from build123d import *

# Parameters (mm, degrees)
SCHIZZO1_R                    = 8
ESTRUSIONE_ESTRUSIONE1_DEPTH  = 30
SCHIZZO2_R                    = 2.5
TAGLIO_ESTRUSIONE1_DEPTH      = 33.062439084
SCHIZZO3_R                    = 4
TAGLIO_ESTRUSIONE2_DEPTH      = 15
TAGLIO_ESTRUSIONE3_DEPTH      = 33.062439084
TAGLIO_ESTRUSIONE3_DEPTH_BACK = 33.062439084
SCHIZZO4_R                    = 1.25


with BuildPart() as part:
    # Schizzo1 → Estrusione-Estrusione1 (new body)
    with BuildSketch(Plane.XY):
        Circle(SCHIZZO1_R)
    extrude(amount=ESTRUSIONE_ESTRUSIONE1_DEPTH)

    # Schizzo2 → Taglio-Estrusione1 (cut, through all)
    with BuildSketch(Plane.XY.offset(30)):
        Circle(SCHIZZO2_R)
    extrude(amount=-TAGLIO_ESTRUSIONE1_DEPTH, mode=Mode.SUBTRACT)

    # Schizzo3 → Taglio-Estrusione2 (cut)
    with BuildSketch(Plane.XY.offset(30)):
        Circle(SCHIZZO3_R)
    extrude(amount=-TAGLIO_ESTRUSIONE2_DEPTH, mode=Mode.SUBTRACT)

    # Schizzo4 → Taglio-Estrusione3 (cut, two sides: drawn at the far end of the back side and taken through both)
    with BuildSketch(Plane(origin=(0, 0, 0), x_dir=(0, 0, -1), z_dir=(1, 0, 0)).offset(-TAGLIO_ESTRUSIONE3_DEPTH_BACK)):
        with Locations((-26, 0)):
            Circle(SCHIZZO4_R)
        with Locations((-4, 0)):
            Circle(SCHIZZO4_R)
    extrude(amount=TAGLIO_ESTRUSIONE3_DEPTH + TAGLIO_ESTRUSIONE3_DEPTH_BACK, mode=Mode.SUBTRACT)


solid = part.part
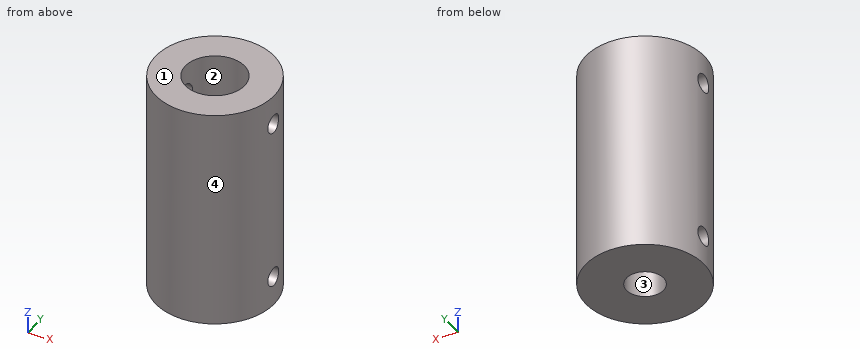
Build history of the part. All positions in model axes, mm. Face numbers are marked on the shaded views. Give positions to 0.01 mm unless a question says otherwise; leave off trailing zeros. Order: outer loops, then holes, each group sorted by start corner. A loop starts at its lowest first (then second) coordinate and runs counter-clockwise, first axis right, second up. Notation, with made-up numbers: M -37,-40 L -26,-40 A26 ccw -26,-12 Z; hole C 73.5,11.5 d5. An arc over 180 degrees is marked long. Use one line per item in the form item = value.
Q1. Pull direction X, two halves, no side cores. Call the marked faces 1, 2, 3 and 4: released by +X, released by -X, zero draft, split by the parting line, or undercut.
Conclusion:
face_1 = zero draft
face_2 = undercut
face_3 = undercut
face_4 = split by the parting line
Q2. Slice it at A-A, the plane y = 0. Write the cut outline in (x, z).
Conclusion:
outline = M -8,0 L -2.5,0 L -2.5,2.75 L -8,2.75 Z; M -8,5.25 L -2.5,5.25 L -2.5,15 L -4,15 L -4,24.75 L -8,24.75 Z; M -8,27.25 L -4,27.25 L -4,30 L -8,30 Z; M 2.5,0 L 8,0 L 8,2.75 L 2.5,2.75 Z; M 2.5,5.25 L 8,5.25 L 8,24.75 L 4,24.75 L 4,15 L 2.5,15 Z; M 4,27.25 L 8,27.25 L 8,30 L 4,30 Z
Q3. Pin check, flat tips, straight feed: P1, Ø3, axis at y = 3.5, z = 9.5, coming from the +X side; P2, Ø7, axis at x = 0, y = 0, coming from the +Z side; P3, Ø1.5, axis at x = 6, z = 8, coming from the -Y side. Stop position of each tip, or through.
Conclusion:
P1 = 7.75
P2 = 15
P3 = -6.04
Q4. Slice it at B-B, the plane x = 0. Write the cut outline in (y, z), and give its area (3 significant figures).
Conclusion:
outline = M -8,0 L -2.5,0 L -2.5,15 L -4,15 L -4,30 L -8,30 Z; M 2.5,0 L 8,0 L 8,30 L 4,30 L 4,15 L 2.5,15 Z
area = 285 mm2
Q5. Slice it at D-D, the plane y = 2. Write the cut outline in (x, z), and give its area (3 significant figures).
Conclusion:
outline = M -7.75,0 L -1.5,0 L -1.5,15 L -3.46,15 L -3.46,30 L -7.75,30 Z; M 1.5,0 L 7.75,0 L 7.75,30 L 3.46,30 L 3.46,15 L 1.5,15 Z
area = 316 mm2
Q6. Wall check: probe 1 along X at (y, z) = (0, 22); probe 2 along Z at (x, y) = (1.5, 3.5); probe 3 along Y at (x, z) = (-1, 6.5). Give the ranges that are in metal, low to high.
Conclusion:
probe_1 = -8 to -4, 4 to 8
probe_2 = 0 to 15
probe_3 = -7.94 to -2.29, 2.29 to 7.94
Q7. Slice it at C-C, the plane z = 4. Write the cut outline in (x, y), and give its area (3 significant figures).
Conclusion:
outline = M -7.9,-1.25 A8 ccw 7.9,-1.25 L 2.17,-1.25 A2.5 cw -2.17,-1.25 Z; M -7.9,1.25 L -2.17,1.25 A2.5 cw 2.17,1.25 L 7.9,1.25 A8 ccw Z
area = 154 mm2
